Geometry: final body of the model. Coordinates: model frame, mm. Face numbers are marked on the shaded views. A direction names the side the tool comes from. Give positions to 0.01 mm unless a question says otherwise; leave off trailing zeros. Write each loop counter-clockwise with the first axis right and the second up, starting at its lowest first coordinate (ties: lowest second). Pieces come first, ordered by that corner, then holes.
Q1. Reachability of the marked faces 5, 6 and 7 from +Z, -Z, +X, -X, +Y, -Y: full face, straight path, thin tool, end or side. Return the list, or none.
Q2. Pin query (flat end, axial travel): pin 1 (5 mm diameter, centred on x = -1.5, z = 18.5, fed in from +Y); pin 2 (8 mm diameter, centred on y = 40, z = 15, fed in from +X); pin 3 (2 mm diameter, centred on y = 33.5, z = 4.5, fed in from +X). Return the tip coordinate at first contact, or that it passes through.
Q3. Draft query along X for the marked faces 1, 2, 3 and 4. Return one class per face: pulls with the +X half, pulls with the -X half, needs draft (parallel to the pull), parting line crosses it, or undercut.
Q4. Cut plane B-B on z = 16.5. Return the cut outline in (x, y), plus the area to 3 significant figures.
Q5. Cut plane C-C on x = -1.25. Return the cut outline in (y, z).
Q6. Cut plane A-A on y = 1. Return the cut outline in (x, z), plus the area to 3 significant figures.
Q7. Cut plane D-D on y = 16. Return the cut outline in (x, z).
Q8. Line query: L1, parallel to X at y = 6.5, z = 23.5; L2, parallel to X at y = 11, z = 24.25; L3, parallel to Y at x = 9, z = 11. Output: solid intervals per line, ascending.
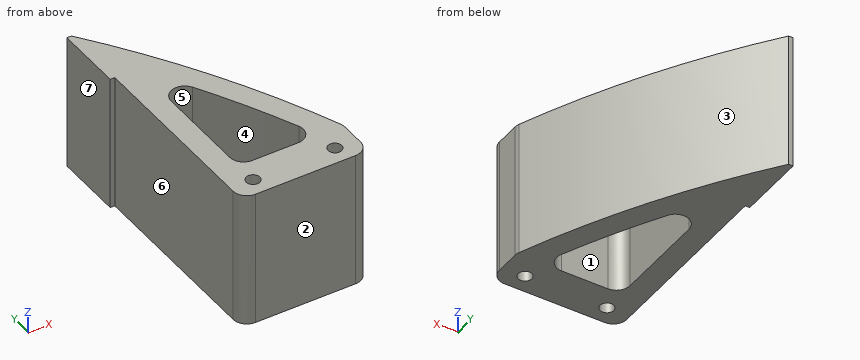
```python
from build123d import *

# Parameters (mm, degrees)
SKETCH_1_W          = 1
SKETCH_1_H          = 15
SKETCH_1_W_2        = 28
SKETCH_1_H_2        = 12
SKETCH_1_R          = 1.5
EXTRUDE_1_DEPTH     = 30
FILLET_1_R          = 3
CUT_EXTRUDE_1_DEPTH = 66.276335681
FILLET_2_R          = 3


with BuildPart() as part:
    # 草图1 → 凸台-拉伸1 (new body)
    # profile 1 of 3: a face of its own
    with BuildSketch(Plane.XY):
        with BuildLine():
            Line((-14, 41), (-14, 6))
            Line((-14, 6), (-9, 6))
            Line((-9, 6), (-9, 40.097477255))
            ThreePointArc((-9, 40.097477255), (0.609436103, 23.461990889), (8.619401339, 6))
            Line((8.619401339, 6), (14, 6))
            ThreePointArc((14, 6), (1.713554205, 31.959590355), (-14, 56))
            Line((-14, 56), (-14, 41))
        make_face()
    # profile 2 of 3: a face of its own
    with BuildSketch(Plane.XY):
        with Locations((-14.5, 48.5)):
            Rectangle(SKETCH_1_W, SKETCH_1_H)
    # profile 3 of 3: a face of its own
    with BuildSketch(Plane.XY):
        Rectangle(SKETCH_1_W_2, SKETCH_1_H_2)
        with Locations((-9, 1)):
            Circle(SKETCH_1_R, mode=Mode.SUBTRACT)
        with Locations((9, 1)):
            Circle(SKETCH_1_R, mode=Mode.SUBTRACT)
    extrude(amount=EXTRUDE_1_DEPTH)

    # 圆角1
    fillet_1_edges = [part.edges().sort_by_distance(p)[0] for p in [
        (-9, 6, 15),
        (8.619401339, 6, 15),
        (-9, 40.097477255, 15),
        (14, -6, 15),
        (-14, -6, 15),
    ]]
    fillet(fillet_1_edges, radius=FILLET_1_R)

    # 草图2 → 切除-拉伸1 (cut, through all)
    with BuildSketch(Plane.XY.offset(30)):
        with BuildLine():
            Line((-14, -3), (14, -3))
            ThreePointArc((14, -3), (13.121320344, -5.121320344), (11, -6))
            Line((11, -6), (-11, -6))
            ThreePointArc((-11, -6), (-13.121320344, -5.121320344), (-14, -3))
        make_face()
    extrude(amount=-CUT_EXTRUDE_1_DEPTH, mode=Mode.SUBTRACT)

    # 圆角2
    fillet_2_edges = [part.edges().sort_by_distance(p)[0] for p in [
        (14, 6, 15),
        (14, -3, 15),
        (-14, -3, 15),
    ]]
    fillet(fillet_2_edges, radius=FILLET_2_R)


solid = part.part
```
Data:
1. face 5: +Z, -Z
1. face 6: +Z, -Z, -X, -Y
1. face 7: +Z, -Z, -X, +Y, -Y
2. pin 1: stops at y = 41.55
2. pin 2: stops at x = -0.61
2. pin 3: stops at x = 1.41
3. face 1: undercut
3. face 2: needs draft
3. face 3: pulls with the +X half
3. face 4: undercut
4. outline: (-15, 41) - (-14, 41) - (-14, 0) arc R3 ccw to (-11, -3) - (11, -3) arc R3 ccw to (14, 0) - (14, 5.43) arc R3 ccw to (13.79, 6.53) arc R210 ccw to (-14, 56) - (-15, 56) - close; hole circle Ø3 at (-9, 1); hole (-9, 9) arc R3 ccw to (-6, 6) - (4.12, 6) arc R3 ccw to (6.88, 10.18) arc R205 ccw to (-3.39, 30.83) arc R3 ccw to (-9, 29.35) - close; hole circle Ø3 at (9, 1)
4. area: 728 mm2
5. outline: (-3, 0) - (6, 0) - (6, 30) - (-3, 30) - close; (26.98, 0) - (37.08, 0) - (37.08, 30) - (26.98, 30) - close
6. outline: (-14, 0) - (-10.5, 0) - (-10.5, 30) - (-14, 30) - close; (-7.5, 0) - (7.5, 0) - (7.5, 30) - (-7.5, 30) - close; (10.5, 0) - (14, 0) - (14, 30) - (10.5, 30) - close
6. area: 660 mm2
7. outline: (-14, 0) - (-9, 0) - (-9, 30) - (-14, 30) - close; (4.28, 0) - (9.78, 0) - (9.78, 30) - (4.28, 30) - close
8. L1: x = -14 to -7.66, 5.78 to 13.8
8. L2: x = -14 to -9, 6.53 to 11.97
8. L3: y = -3 to -0.5, 2.5 to 17.7
